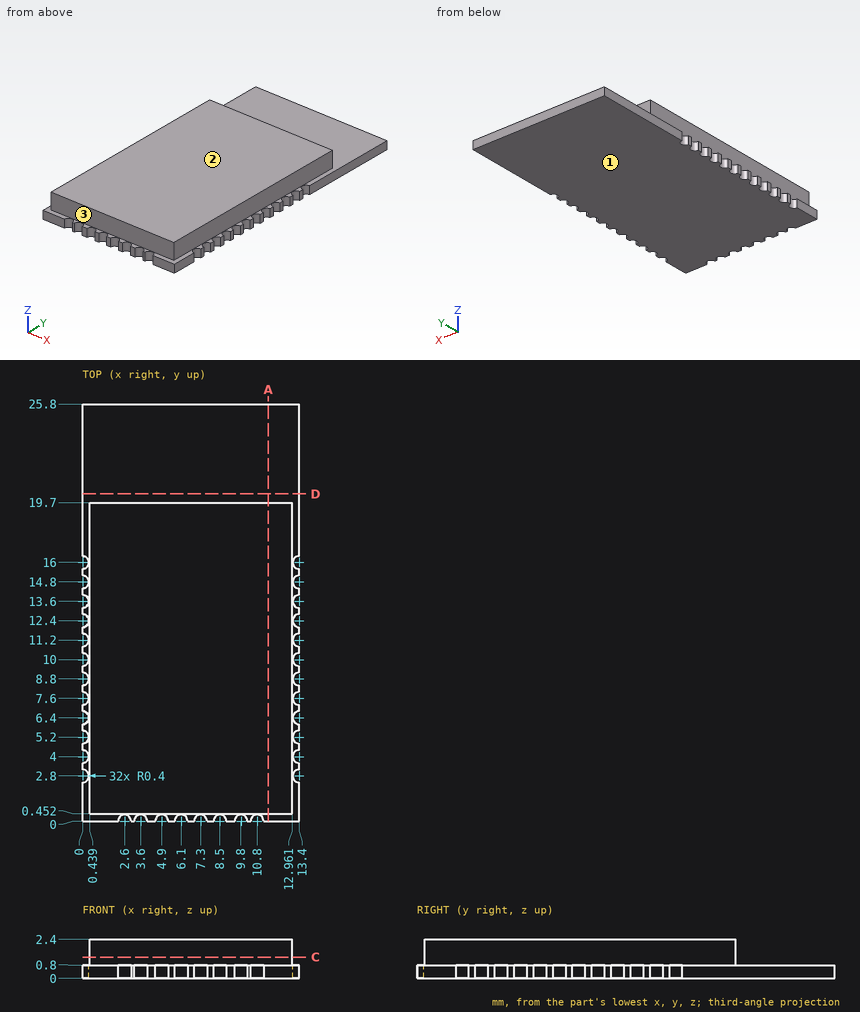
Verification items for this drawing (mm, ordinates from the low corner). Coordinates: 2 decimals unless noted, no trailing zeros. Order: outer loops, then holes, each group sorted by start corner. A loop starts at its lowest first (then second) coordinate and runs counter-clockwise, first axis right, second up. Notation, with made-up numbers: (5, 74.25) -> (49, 74.25) arc R23 cw to (49, 96.25) -> close; hole circle Ø7 at (25.5, -14.75). An arc over 180 degrees is marked (long way). Put each result on its own line as item: value. Start each with the question number.
1. Cross-section at A-A, the plane x = 11.5. Record the boundary of the cut face in (y, z).
2. Go/stop test with flat-tipped pins: pin 1 Ø1.5 at (x, y) = (11.5, 5.5) entering from -Z; pin 2 Ø4 at (x, y) = (10.5, 22) entering from +Z; pin 3 Ø1.3 at (y, z) = (6, 2) entering from +X. Record where each tip stops, or that it passes through.
3. Cross-section at D-D, the plane y = 20.25. Record the boundary of the cut face in (x, z).
4. Cross-section at C-C, the plane z = 1.3. Record the boundary of the cut face in (x, y), then the cut area to 3 significant figures.
5. Mould release check, pull along Z, two halves, no side actions. Record for the marked faces 1, 2 and 3: released by +Z, released by -Z, zero draft, split by the parting line, or undercut.
6. Material ranges on L1, parallel to Y at x = 3.75, z = 1.65; L2, parallel to Z at x = 12, y = 20.75; L3, parallel to X at y = 3.5, z = 2, recorded low to high. Write a range as [from, to].
Computed:
1. outline: (0, 0) -> (25.8, 0) -> (25.8, 0.8) -> (19.7, 0.8) -> (19.7, 2.4) -> (0.45, 2.4) -> (0.45, 0.8) -> (0, 0.8) -> close
2. pin 1: z = 0
2. pin 2: z = 0.8
2. pin 3: x = 12.96
3. outline: (0, 0) -> (13.4, 0) -> (13.4, 0.8) -> (0, 0.8) -> close
4. outline: (0.44, 0.45) -> (12.96, 0.45) -> (12.96, 19.7) -> (0.44, 19.7) -> close
4. area: 241 mm2
5. face 1: released by -Z
5. face 2: released by +Z
5. face 3: zero draft
6. L1: [0.45, 19.7]
6. L2: [0, 0.8]
6. L3: [0.44, 12.96]
